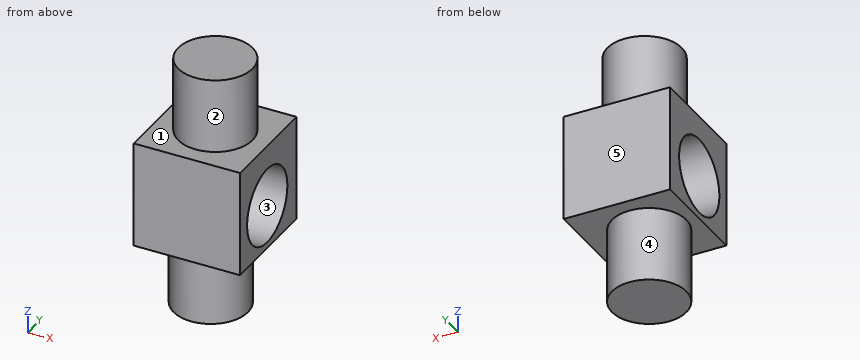
```python
from build123d import *

# Parameters (mm, degrees)
F0_W     = 100
F0_H     = 100
F1_DEPTH = 100
F2_R     = 35
F3_DEPTH = 70
F4_R     = 35
F5_DEPTH = 70
F6_R     = 35.831908
F7_DEPTH = 100.001


with BuildPart() as f1:
    # F0 (on Front) → F1 (new body)
    with BuildSketch(Plane.XZ):
        with Locations((50, 50)):
            Rectangle(F0_W, F0_H)
    extrude(amount=F1_DEPTH)

    # F2 (on face) → F3 (join)
    with BuildSketch(Plane.XY.offset(100)):
        with Locations((50.003812, -49.382195)):
            Circle(F2_R)
    extrude(amount=F3_DEPTH)

    # F4 (on face) → F5 (join)
    with BuildSketch(Plane(origin=(0, 0, 0), x_dir=(1, 0, 0), z_dir=(0, 0, -1))):
        with Locations((45.392986, 48.75914)):
            Circle(F4_R)
    extrude(amount=F5_DEPTH)

    # F6 (on face) → F7 (cut, through all)
    with BuildSketch(Plane.YZ.offset(100)):
        with Locations((-51.767617, 41.582473)):
            Circle(F6_R)
    extrude(amount=-F7_DEPTH, mode=Mode.SUBTRACT)


solid = f1.part
```
Here's how the part is built. I have some questions about the finished solid (model axes, mm). Face numbers are marked on the shaded views. A direction names the side the tool comes from. Give positions to 0.01 mm unless a question says otherwise; leave off trailing zeros. Loops run counter-clockwise (first coordinate to the right, second up) from the corner with the lowest first, then second, coordinate; pieces in that order, holes last. Notation, with made-up numbers: M -1.5,87 L 22.5,87 A15 ccw 22.5,104 Z; hole C 75,-31.75 d1. An arc over 180 degrees is marked long. Return JSON: item names as keys, results as strings.
Item 1: Imagine slicing it at D-D on y = -28. List the corners of the cut face in (x, z) for me.
A:
{"outline": "M 0,0 L 17.21,0 L 17.21,-70 L 73.57,-70 L 73.57,0 L 100,0 L 100,14.77 L 0,14.77 Z; M 0,68.4 L 100,68.4 L 100,100 L 77.71,100 L 77.71,170 L 22.29,170 L 22.29,100 L 0,100 Z"}
Item 2: Imagine slicing it at C-C on x = 29. List the corners of the cut face in (y, z) for me.
A:
{"outline": "M -100,0 L -79.68,0 L -79.68,-70 L -17.84,-70 L -17.84,0 L 0,0 L 0,100 L -21.39,100 L -21.39,170 L -77.38,170 L -77.38,100 L -100,100 Z; hole C -51.77,41.58 d71.66"}
Item 3: Thinking about a two-plate mould opening in Z: for the marked faces 1, 2 and 3, which applies, released by +Z, released by -Z, zero draft, split by the parting line, or undercut?
A:
{"face 1": "released by +Z", "face 2": "zero draft", "face 3": "undercut"}
Item 4: Imagine slicing it at A-A on y = -56.5. List the corners of the cut face in (x, z) for me.
A:
{"outline": "M 0,0 L 11.26,0 L 11.26,-70 L 79.53,-70 L 79.53,0 L 100,0 L 100,6.06 L 0,6.06 Z; M 0,77.1 L 100,77.1 L 100,100 L 84.27,100 L 84.27,170 L 15.74,170 L 15.74,100 L 0,100 Z"}
Item 5: On a 3-axis mill with a long thin cutter (end or side, diameter ignored), from which of +Z, -Z, +X, -X, +Y, -Y can I reach the whole of each face in a straight line? I mean the marked faces 4 and 5. Say none if no direction works.
A:
{"face 4": "-Z", "face 5": "+Z, -Z, +X, -X, +Y"}
Item 6: I'm going to push flat-ended pins straight in: pin 1 Ø5 at (x, z) = (51, -33.5) entering from +Y; pin 2 Ø5 at (x, z) = (73, 118.5) entering from +Y; pin 3 Ø6 at (y, z) = (-50.5, -19) entering from +X. Where does each tip first touch, or does it pass through?
A:
{"pin 1": "stops at y = -13.9", "pin 2": "stops at y = -21.01", "pin 3": "stops at x = 80.39"}
Item 7: Imagine slicing it at B-B on z = 9.5. List the corners of the cut face in (x, y) for me.
A:
{"outline": "M 0,-100 L 100,-100 L 100,-67.73 L 0,-67.73 Z; M 0,-35.81 L 100,-35.81 L 100,0 L 0,0 Z"}
Item 8: Please list where these lines run through material, in increasing order: line 1 (Z direction, x = 93, y = -50.5); line 2 (Z direction, x = 80.5, y = -88); line 3 (Z direction, x = 93.5, y = -33.5).
A:
{"line 1": "z = 0 to 5.77, 77.39 to 100", "line 2": "z = 0 to 100", "line 3": "z = 0 to 10.76, 72.41 to 100"}
